from build123d import *

# Parameters (mm, degrees)
F0_W            = 170
F0_H            = 76
F1_DEPTH        = 6
F2_W            = 164.4
F2_H            = 70.4
F3_DEPTH        = 3
F4_R            = 3.5
F5_DEPTH        = 7
F6_R            = 4
F7_DEPTH        = 2.8
F8_W            = 166
F8_H            = 72
F8_W_2          = 163.2
F8_H_2          = 69.2
F9_DEPTH        = 2
F10_R           = 3.5
F11_DEPTH       = 10
F12_R           = 0.5
F13_DEPTH       = 0.5
F14_R           = 0.5
F15_DEPTH       = 0.5
F17_D           = 3
F17_DEPTH       = 2.5
F17_CSINK_D     = 6.72
F17_CSINK_ANGLE = 90
F17_TIP         = 0.9012909285
F18_T1_DEPTH    = 13.5
F18_T3_DEPTH    = 66
F18_T5_DEPTH    = 160
F18_S9_W        = 5
F18_S9_H        = 5
F18_T10_DEPTH   = 5
F18_S15_W       = 5
F18_S15_H       = 5
F18_T16_DEPTH   = 5
F18_S21_W       = 5
F18_S21_H       = 5
F18_T22_DEPTH   = 5
F18_S27_W       = 5
F18_S27_H       = 5
F18_T28_DEPTH   = 5


# Not quite as in the source:
# - a fillet or chamfer that OpenCascade refuses, or shapes differently, is made with other operations: its cross-section is extruded or revolved along the edge and cut away or added


with BuildPart() as f1:
    # F0 (on Top) → F1 (new body)
    with BuildSketch(Plane.XY):
        with Locations((85, 38)):
            Rectangle(F0_W, F0_H)
    extrude(amount=F1_DEPTH)

    # F2 (on face) → F3 (cut)
    with BuildSketch(Plane.XY.offset(6)):
        with Locations((85, 38)):
            Rectangle(F2_W, F2_H)
    extrude(amount=-F3_DEPTH, mode=Mode.SUBTRACT)

    # F4 (on face) → F5 (join)
    with BuildSketch(Plane.XY.offset(3)):
        with Locations((22.8, 68.5)):
            Circle(F4_R)
        with Locations((22.8, 7.5)):
            Circle(F4_R)
        with Locations((80.3, 68.5)):
            Circle(F4_R)
        with Locations((80.3, 7.5)):
            Circle(F4_R)
        with Locations((116.8, 68.5)):
            Circle(F4_R)
        with Locations((145.8, 52.5)):
            Circle(F4_R)
        with Locations((116.8, 23.5)):
            Circle(F4_R)
        with Locations((145.8, 7.5)):
            Circle(F4_R)
    extrude(amount=F5_DEPTH)

    # F6 (on face) → F7 (cut, through all)
    with BuildSketch(Plane(origin=(0, 0, 0), x_dir=(0, -1, 0), z_dir=(-1, 0, 0))):
        with Locations((-57, 18)):
            Circle(F6_R)
        with Locations((-19, 18)):
            Circle(F6_R)
    extrude(amount=-F7_DEPTH, mode=Mode.SUBTRACT)

    # F8 (on face) → F9 (cut)
    with BuildSketch(Plane.XY.offset(6)):
        with Locations((85, 38)):
            Rectangle(F8_W, F8_H)
        with Locations((84.6, 37.6)):
            Rectangle(F8_W_2, F8_H_2, mode=Mode.SUBTRACT)
    extrude(amount=-F9_DEPTH, mode=Mode.SUBTRACT)

    # F10 (on face) → F11 (join)
    with BuildSketch(Plane.XY.offset(3)):
        with Locations((8, 68.2)):
            Circle(F10_R)
        with Locations((8, 7.8)):
            Circle(F10_R)
        with Locations((162, 7.8)):
            Circle(F10_R)
        with Locations((162, 68.2)):
            Circle(F10_R)
    extrude(amount=F11_DEPTH)

    # F12 (on face) → F13 (cut)
    with BuildSketch(Plane.XY.offset(13)):
        with Locations((8, 67.8)):
            Circle(F12_R)
        with Locations((8, 7.8)):
            Circle(F12_R)
        with Locations((162, 7.8)):
            Circle(F12_R)
        with Locations((162, 67.8)):
            Circle(F12_R)
    extrude(amount=-F13_DEPTH, mode=Mode.SUBTRACT)

    # F14 (on face) → F15 (cut)
    with BuildSketch(Plane.XY.offset(10)):
        with Locations((22.8, 68.5)):
            Circle(F14_R)
        with Locations((22.8, 7.5)):
            Circle(F14_R)
        with Locations((80.3, 68.5)):
            Circle(F14_R)
        with Locations((80.3, 7.5)):
            Circle(F14_R)
        with Locations((116.8, 68.5)):
            Circle(F14_R)
        with Locations((147.8, 52.5)):
            Circle(F14_R)
        with Locations((116.8, 23.5)):
            Circle(F14_R)
        with Locations((147.8, 7.5)):
            Circle(F14_R)
    extrude(amount=-F15_DEPTH, mode=Mode.SUBTRACT)

    # F17
    with Locations(Plane(origin=(0, 0, 0), x_dir=(1, 0, 0), z_dir=(0, 0, -1))):
        with Locations((8, -8), (8, -68), (162, -68), (162, -8)):
            CounterSinkHole(F17_D / 2, F17_CSINK_D / 2, depth=F17_DEPTH, counter_sink_angle=F17_CSINK_ANGLE)
            with Locations((0, 0, -(F17_DEPTH + F17_TIP / 2))):  # 118° drill point
                Cone(0, F17_D / 2, F17_TIP, mode=Mode.SUBTRACT)

    # F18: fillet of radius 5 on 8 edges, made by hand

    # F18_s2 → F18_t1 (cut)
    with BuildSketch(Plane.XY.offset(5)):
        with BuildLine():
            ThreePointArc((165, 76), (168.5355339059, 74.5355339059), (170, 71))
            Line((170, 71), (170, 76))
            Line((170, 76), (165, 76))
        make_face()
        with BuildLine():
            ThreePointArc((165, 0), (168.5355339059, 1.4644660941), (170, 5))
            Line((170, 5), (170, 0))
            Line((170, 0), (165, 0))
        make_face()
        with BuildLine():
            ThreePointArc((0, 71), (1.4644660941, 74.5355339059), (5, 76))
            Line((5, 76), (0, 76))
            Line((0, 76), (0, 71))
        make_face()
        with BuildLine():
            ThreePointArc((0, 5), (1.4644660941, 1.4644660941), (5, 0))
            Line((5, 0), (0, 0))
            Line((0, 0), (0, 5))
        make_face()
    extrude(amount=F18_T1_DEPTH, mode=Mode.SUBTRACT)

    # F18_s4 → F18_t3 (cut)
    with BuildSketch(Plane.XZ.offset(-71)):
        with BuildLine():
            ThreePointArc((165, 0), (168.5355339059, 1.4644660941), (170, 5))
            Line((170, 5), (170, 0))
            Line((170, 0), (165, 0))
        make_face()
        with BuildLine():
            ThreePointArc((0, 5), (1.4644660941, 1.4644660941), (5, 0))
            Line((5, 0), (0, 0))
            Line((0, 0), (0, 5))
        make_face()
    extrude(amount=F18_T3_DEPTH, mode=Mode.SUBTRACT)

    # F18_s6 → F18_t5 (cut)
    with BuildSketch(Plane.YZ.offset(5)):
        with BuildLine():
            ThreePointArc((76, 5), (74.5355339059, 1.4644660941), (71, 0))
            Line((71, 0), (76, 0))
            Line((76, 0), (76, 5))
        make_face()
        with BuildLine():
            ThreePointArc((0, 5), (1.4644660941, 1.4644660941), (5, 0))
            Line((5, 0), (0, 0))
            Line((0, 0), (0, 5))
        make_face()
    extrude(amount=F18_T5_DEPTH, mode=Mode.SUBTRACT)


with BuildPart() as f18_tool8:
    # F18_s9 → F18_t10 (new body)
    with BuildSketch(Plane.XZ.offset(-71)):
        with Locations((167.5, 2.5)):
            Rectangle(F18_S9_W, F18_S9_H)
    extrude(amount=-F18_T10_DEPTH)

    # F18_s11 → F18_t12 (revolve, cut)
    with BuildSketch(Plane(origin=(165, 71, 5), x_dir=(-0.7071067812, 0, 0.7071067812), z_dir=(-0.7071067812, 0, -0.7071067812))):
        with BuildLine():
            ThreePointArc((0, -5), (5, 0), (0, 5))
            Line((0, 5), (0, -5))
        make_face()
    revolve(axis=Axis((165, 71, 5), (0, 1, 0)), mode=Mode.SUBTRACT)


with BuildPart() as f1_1:
    add(f1.part)

    # F18_t7: cut F18_tool8
    add(f18_tool8.part, mode=Mode.SUBTRACT)


with BuildPart() as f18_tool14:
    # F18_s15 → F18_t16 (new body)
    with BuildSketch(Plane.XZ.offset(-5)):
        with Locations((167.5, 2.5)):
            Rectangle(F18_S15_W, F18_S15_H)
    extrude(amount=F18_T16_DEPTH)

    # F18_s17 → F18_t18 (revolve, cut)
    with BuildSketch(Plane(origin=(165, 5, 5), x_dir=(-0.7071067812, 0, 0.7071067812), z_dir=(0.7071067812, 0, 0.7071067812))):
        with BuildLine():
            ThreePointArc((0, -5), (5, 0), (0, 5))
            Line((0, 5), (0, -5))
        make_face()
    revolve(axis=Axis((165, 5, 5), (0, -1, 0)), mode=Mode.SUBTRACT)


with BuildPart() as f1_2:
    add(f1_1.part)

    # F18_t13: cut F18_tool14
    add(f18_tool14.part, mode=Mode.SUBTRACT)


with BuildPart() as f18_tool20:
    # F18_s21 → F18_t22 (new body)
    with BuildSketch(Plane.YZ.offset(5)):
        with Locations((73.5, 2.5)):
            Rectangle(F18_S21_W, F18_S21_H)
    extrude(amount=-F18_T22_DEPTH)

    # F18_s23 → F18_t24 (revolve, cut)
    with BuildSketch(Plane(origin=(5, 71, 5), x_dir=(0, -0.7071067812, 0.7071067812), z_dir=(0, -0.7071067812, -0.7071067812))):
        with BuildLine():
            ThreePointArc((0, -5), (5, 0), (0, 5))
            Line((0, 5), (0, -5))
        make_face()
    revolve(axis=Axis((5, 71, 5), (-1, 0, 0)), mode=Mode.SUBTRACT)


with BuildPart() as f1_3:
    add(f1_2.part)

    # F18_t19: cut F18_tool20
    add(f18_tool20.part, mode=Mode.SUBTRACT)


with BuildPart() as f18_tool26:
    # F18_s27 → F18_t28 (new body)
    with BuildSketch(Plane.YZ.offset(5)):
        with Locations((2.5, 2.5)):
            Rectangle(F18_S27_W, F18_S27_H)
    extrude(amount=-F18_T28_DEPTH)

    # F18_s29 → F18_t30 (revolve, cut)
    with BuildSketch(Plane(origin=(5, 5, 5), x_dir=(0, 0.7071067812, 0.7071067812), z_dir=(0, -0.7071067812, 0.7071067812))):
        with BuildLine():
            ThreePointArc((0, -5), (5, 0), (0, 5))
            Line((0, 5), (0, -5))
        make_face()
    revolve(axis=Axis((5, 5, 5), (-1, 0, 0)), mode=Mode.SUBTRACT)


with BuildPart() as f1_4:
    add(f1_3.part)

    # F18_t25: cut F18_tool26
    add(f18_tool26.part, mode=Mode.SUBTRACT)


solid = f1_4.part
Source: CAD feature listing. Evaluate the final solid. Frame: model axes, mm. A direction names the side the tool comes from. Coordinates: 2 decimals unless noted, no trailing zeros. Order: outer loops, then holes, each group sorted by start corner. A loop starts at its lowest first (then second) coordinate and runs counter-clockwise, first axis right, second up. Notation, with made-up numbers: M 83,5.5 L 134,5.5 A25 ccw 134,21.5 Z; hole C 41.25,38.25 d11. An arc over 180 degrees is marked long. Write each question's results on one line, items separated by ' | '. Start each with the question number.
Item 1: Line query: probe 1 along Y at (x, z) = (8.5, 7.25); probe 2 along X at (y, z) = (10, 9); probe 3 along Y at (x, z) = (81, 4.25). Output: solid intervals per line, ascending.
Item 2: Set-up query: faces 1 (the face through (7.194, 66.735, 2.184)), 2 (the face through (22.8, 6.8, 10)), 3 (the face through (165.233, 66.859, 7.93)). Return all of +Z, -Z, +X, -X, +Y, -Y with unobstructed straight access to the full face (end or side cutting, diameter ignored); none if empty.
Item 3: First-contact query: pin 1 Ø3.5 at (x, y) = (145.5, 53.5) entering from +Z; pin 2 Ø23 at (x, y) = (53.5, 29) entering from +Z; pin 3 Ø3.5 at (x, y) = (162, 8) entering from -Z. Flat tips, straight axial feed; report the tip coordinate or a pass-through.
Item 4: Cut plane B-B (y = 45.5). Return loops of the section in (x, z).
Item 5: Draft query along Y for faces 4 (the face through (118, 69, 10)), 5 (the face through (142.303, 7.654, 6.451)), 6 (the face through (168.5, 74.57, 5.49)). Return one class per face: pulls with the +Y half, pulls with the -Y half, needs draft (parallel to the pull), parting line crosses it, or undercut.
Item 6: Cut plane A-A (x = 14.5). Return loops of the section in (y, z).
Checked values:
1) probe 1: y = 4.34 to 11.26, 64.74 to 71.66 | probe 2: x = 5.28 to 10.72, 20.35 to 25.25, 77.85 to 82.75, 143.35 to 148.25, 159.28 to 164.72 | probe 3: y = 0.06 to 2, 4.07 to 10.93, 65.07 to 71.93, 74 to 75.94
2) face 1: -Z | face 2: +Z, +Y, -Y | face 3: +Z
3) pin 1: stops at z = 10 | pin 2: stops at z = 3 | pin 3: stops at z = 1.61
4) outline: M 0,5 A5 ccw 5,0 L 165,0 A5 ccw 170,5 L 170,6 L 168,6 L 168,4 L 167.2,4 L 167.2,3 L 2.8,3 L 2.8,4 L 2,4 L 2,6 L 0,6 Z
5) face 4: needs draft | face 5: undercut | face 6: pulls with the +Y half
6) outline: M 0,5 A5 ccw 5,0 L 71,0 A5 ccw 76,5 L 76,6 L 74,6 L 74,4 L 73.2,4 L 73.2,3 L 2.8,3 L 2.8,4 L 2,4 L 2,6 L 0,6 Z
